The listing builds one solid part. Answer for the finished solid, in the listing's coordinates (mm). A direction names the side the tool comes from. Coordinates: 2 decimals unless noted, no trailing zeros. Order: outer loops, then holes, each group sorted by start corner. A loop starts at its lowest first (then second) coordinate and runs counter-clockwise, first axis right, second up. Notation, with made-up numbers: M 52.5,-21.5 L 60.5,-21.5 A16 cw 60.5,9.5 Z; hole C 44.25,86.25 d8. An arc over 180 degrees is marked long. One line per item, written item: value. Start each with the question number.
Q1. Straight lines are drawn through the part: line 1 along Z through (x, y) = (-22, -10.7); line 2 along X through (y, z) = (0.5, 28); line 3 along X through (y, z) = (-8.5, 15). For each, find the intervals that lie inside material, in ascending order. Write a range as [from, to].
Q2. Determine the mould class of faces 6 (the flat face through (6.5, -11, 15)), 7 (the flat face through (-12.1, -3.9, 0)), 8 (the flat face through (-27, -10, 15)) for opening direction X: pulls with the +X half, pulls with the -X half, needs draft (parallel to the pull), parting line crosses it, or undercut.
Q3. For faces 1 (the flat face through (-17, -3, 15)), 2 (the flat face through (-17, -12, 15)), 3 (the flat face through (-6.5, -11, 15)), 4 (the flat face through (-12.1, -3.9, 30)), 5 (the flat face through (19.7, -7, 14.8)), determine the directions among +Z, -Z, +X, -X, +Y, -Y from which every point of the face is accessible in a straight line to the end or side of a thin tool.
Q4. The part is cut by section B-B on z = 8. Give the vertices of the cut face in (x, y).
Q5. The part is cut by section A-A on x = 22. Give the vertices of the cut face in (y, z), then the cut area to 3 significant figures.
Q6. Each of these flat-tipped pins is pushed along its axis until it touches: pin 1 Ø3.5 at (y, z) = (-2.5, 21) entering from -X; pin 2 Ø1.5 at (x, z) = (-2.5, 18) entering from +Y; pin 3 Ø3 at (x, z) = (-20.5, 17) entering from +Y. Where does it stop, or does it pass through?
Q7. The part is cut by section C-C on y = 7.5. Give the vertices of the cut face in (x, z), then the cut area to 3 significant figures.
Q8. The part is cut by section D-D on x = 0. Give the vertices of the cut face in (y, z).
```python
from build123d import *

# Parameters (mm, degrees)
F0_W      = 10
F0_H      = 5
F1_DEPTH  = 30
F2_R      = 2
F1_FACE_W = 20.5
F1_FACE_H = 30
F3_DEPTH  = 25


with BuildPart() as f1:
    # F0 (on Top) → F1 (new body)
    with BuildSketch(Plane.XY):
        with Locations((-22, -9.5)):
            Rectangle(F0_W, F0_H)
        with Locations((22, -9.5)):
            Rectangle(F0_W, F0_H)
        with BuildLine():
            ThreePointArc((-15.4919333848, -7), (-16.6187073436, -3.5803025332), (-17, 0))
            Line((-17, 0), (-17, -7))
            Line((-17, -7), (-15.4919333848, -7))
        make_face()
        with BuildLine():
            Line((17, -7), (17, 0))
            ThreePointArc((17, 0), (16.6187073436, -3.5803025332), (15.4919333848, -7))
            Line((15.4919333848, -7), (17, -7))
        make_face()
        with BuildLine():
            Line((12.5, 0), (17, 0))
            ThreePointArc((17, 0), (0, 17), (-17, 0))
            Line((-17, 0), (-12.5, 0))
            ThreePointArc((-12.5, 0), (0, 12.5), (12.5, 0))
        make_face()
        with BuildLine():
            Line((-12.5, 0), (-17, 0))
            ThreePointArc((-17, 0), (-16.6187073436, -3.5803025332), (-15.4919333848, -7))
            Line((-15.4919333848, -7), (-10.3561575886, -7))
            ThreePointArc((-10.3561575886, -7), (-11.9520284859, -3.6604665101), (-12.5, 0))
        make_face()
        with BuildLine():
            ThreePointArc((-12.0415945788, -12), (-13.991918758, -9.6553720523), (-15.4919333848, -7))
            Line((-15.4919333848, -7), (-17, -7))
            Line((-17, -7), (-17, -12))
            Line((-17, -12), (-12.0415945788, -12))
        make_face()
        with BuildLine():
            Line((17, -7), (15.4919333848, -7))
            ThreePointArc((15.4919333848, -7), (13.991918758, -9.6553720523), (12.0415945788, -12))
            Line((12.0415945788, -12), (17, -12))
            Line((17, -12), (17, -7))
        make_face()
        with BuildLine():
            ThreePointArc((15.4919333848, -7), (16.6187073436, -3.5803025332), (17, 0))
            Line((17, 0), (12.5, 0))
            ThreePointArc((12.5, 0), (11.9520284859, -3.6604665101), (10.3561575886, -7))
            Line((10.3561575886, -7), (15.4919333848, -7))
        make_face()
        with BuildLine():
            Line((-10.3561575886, -7), (-15.4919333848, -7))
            ThreePointArc((-15.4919333848, -7), (-13.991918758, -9.6553720523), (-12.0415945788, -12))
            Line((-12.0415945788, -12), (-6.5, -12))
            Line((-6.5, -12), (-6.5, -10.677078252))
            ThreePointArc((-6.5, -10.677078252), (-8.6262818341, -9.0463949571), (-10.3561575886, -7))
        make_face()
        with BuildLine():
            ThreePointArc((12.0415945788, -12), (13.991918758, -9.6553720523), (15.4919333848, -7))
            Line((15.4919333848, -7), (10.3561575886, -7))
            ThreePointArc((10.3561575886, -7), (8.6262818341, -9.0463949571), (6.5, -10.677078252))
            Line((6.5, -10.677078252), (6.5, -12))
            Line((6.5, -12), (12.0415945788, -12))
        make_face()
    extrude(amount=F1_DEPTH)

    # F2 (on Front) + F1_face (on face) → F3 (cut)
    with BuildSketch(Plane.XZ):
        with Locations((-22, 15)):
            Circle(F2_R)
        with Locations((22, 15)):
            Circle(F2_R)
    with BuildSketch(Plane(origin=(-16.75, -12, 15), x_dir=(1, 0, 0), z_dir=(0, -1, 0))):
        Rectangle(F1_FACE_W, F1_FACE_H)
        with Locations((33.5, 0)):
            Rectangle(F1_FACE_W, F1_FACE_H)
    extrude(amount=F3_DEPTH, mode=Mode.SUBTRACT)


solid = f1.part
```
Output:
1. line 1: z = [0, 13], [17, 30]
1. line 2: x = [-16.99, -12.49], [12.49, 16.99]
1. line 3: x = [-27, -24], [-20, -9.17], [9.17, 20], [24, 27]
2. face 6: undercut
2. face 7: needs draft
2. face 8: pulls with the -X half
3. face 1: +Z, -Z, -X, +Y
3. face 2: +Z, -Z, +X, -X, -Y
3. face 3: +Z, -Z, -Y
3. face 4: +Z, +X, -X, +Y, -Y
3. face 5: +Z, -Z, +X, +Y
4. outline: M -27,-12 L -6.5,-12 L -6.5,-10.68 A12.5 cw long 6.5,-10.68 L 6.5,-12 L 27,-12 L 27,-7 L 17,-7 L 17,0 A17 ccw -17,0 L -17,-7 L -27,-7 Z
5. outline: M -12,0 L -7,0 L -7,13 L -12,13 Z; M -12,17 L -7,17 L -7,30 L -12,30 Z
5. area: 130 mm^2
6. pin 1: stops at x = -17
6. pin 2: stops at y = 16.91
6. pin 3: stops at y = -7
7. outline: M -15.26,0 L -10,0 L -10,30 L -15.26,30 Z; M 10,0 L 15.26,0 L 15.26,30 L 10,30 Z
7. area: 315 mm^2
8. outline: M 12.5,0 L 17,0 L 17,30 L 12.5,30 Z
